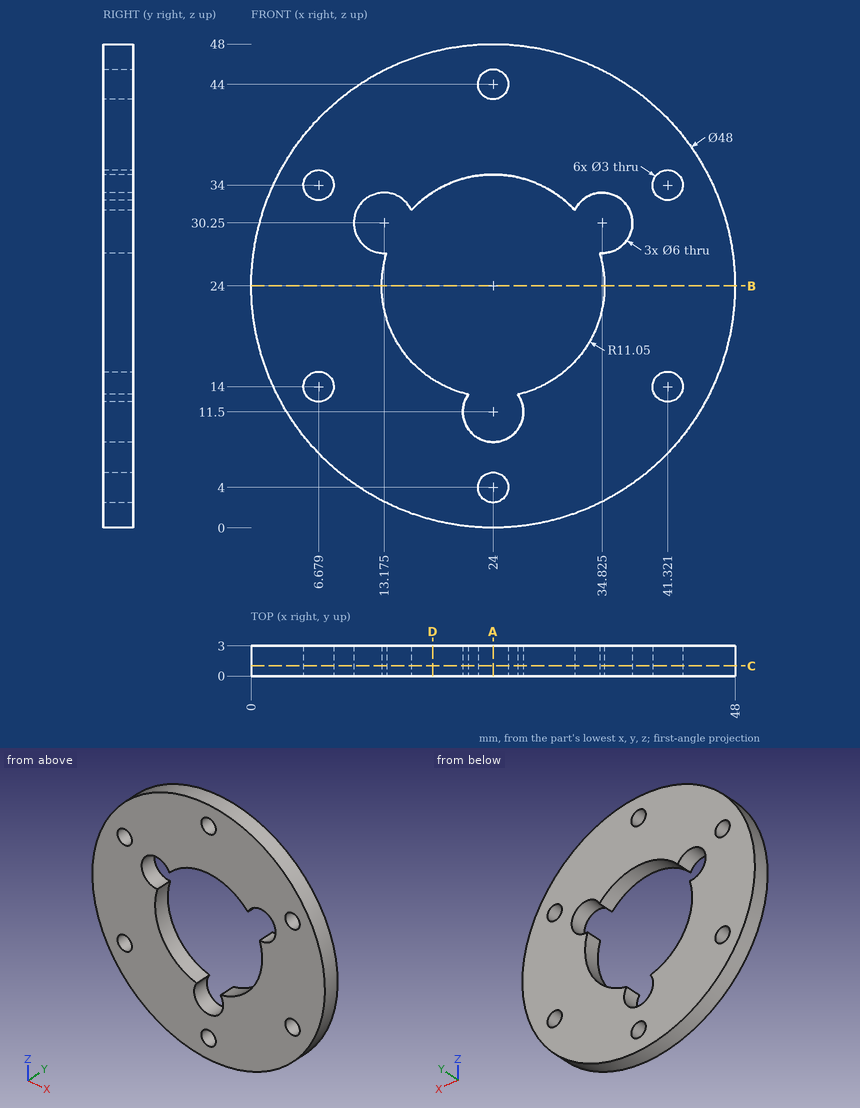
Geometry check sheet. Reference: drawing and pictorial views, mm from the part's lowest x, y, z. Round coordinates to 2 decimals unless told otherwise and drop trailing zeros. Write each loop counter-clockwise with the first axis right and the second up, starting at its lowest first coordinate (ties: lowest second). Pieces come first, ordered by that corner, then holes. Notation, with made-up numbers: (50.5, 50.25) -> (57.5, 50.25) arc R19 cw to (57.5, 76.25) -> close; hole circle Ø8 at (25.5, -23). An arc over 180 degrees is marked (long way). Answer as CSV lines item,"result". Start each with the question number.
1) Section check A-A on x = 24. Enter the section's corners in (y, z).
2) Section check B-B on z = 24. Enter the section's corners in (x, y).
3) Go/stop test with a flat-tipped pin: P1, Ø1, axis at y = 2.5, z = 7, coming from the -X side. Record where the tip stops, or that it passes through.
4) Section check D-D on x = 18. Enter the section's corners in (y, z).
5) Material ranges on line 1 (X direction, y = 0.8, z = 14) (1 decimal); line 2 (Z direction, x = 25, y = 1.85) (1 decimal); line 3 (Z direction, x = 7, y = 0.25) (1 decimal), recorded low to high. Write a range as from..to.
6) Section check C-C on y = 1. State how many separate pieces and enclosed holes the cut face has, and give its area (3 significant figures).
Found:
1,outline,"(0, 0) -> (3, 0) -> (3, 2.5) -> (0, 2.5) -> close; (0, 5.5) -> (3, 5.5) -> (3, 8.5) -> (0, 8.5) -> close; (0, 35.05) -> (3, 35.05) -> (3, 42.5) -> (0, 42.5) -> close; (0, 45.5) -> (3, 45.5) -> (3, 48) -> (0, 48) -> close"
2,outline,"(0, 0) -> (12.95, 0) -> (12.95, 3) -> (0, 3) -> close; (35.05, 0) -> (48, 0) -> (48, 3) -> (35.05, 3) -> close"
3,P1,"stops at x = 6.57"
4,outline,"(0, 0.76) -> (3, 0.76) -> (3, 14.72) -> (0, 14.72) -> close; (0, 33.28) -> (3, 33.28) -> (3, 47.24) -> (0, 47.24) -> close"
5,line 1,"x = 2.2..5.2, 8.2..19.3, 28.7..39.8, 42.8..45.8"
5,line 2,"z = 0..2.9, 5.1..8.7, 35..42.9, 45.1..48"
5,line 3,"z = 7.1..12.5, 15.5..32.5, 35.5..40.9"
6,separate pieces,"1"
6,enclosed holes,"7"
6,area,"1,310 mm^2"
